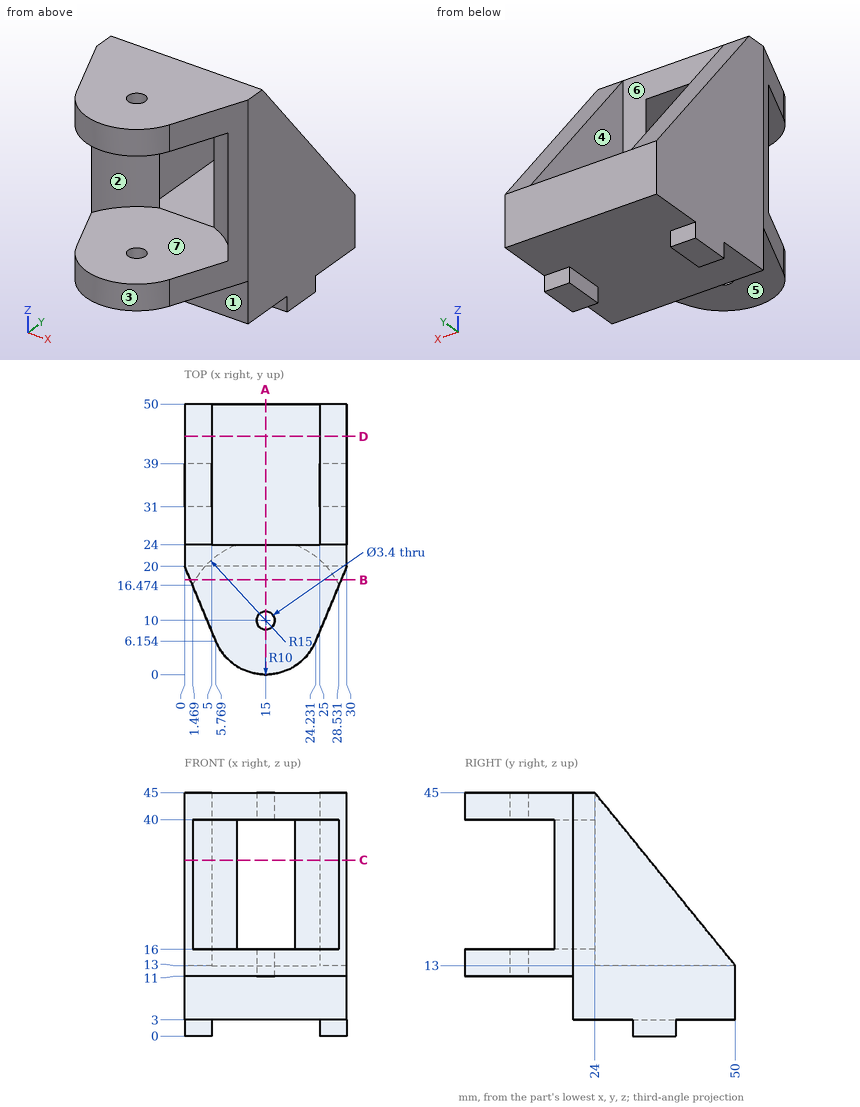
Verification items for this drawing (mm, ordinates from the low corner). A direction names the side the tool comes from. Give positions to 0.01 mm unless a question says otherwise; leave off trailing zeros. Loops run counter-clockwise (first coordinate to the right, second up) from the corner with the lowest first, then second, coordinate; pieces in that order, holes last. Notation, with made-up numbers: M -35,20 L 0,20 A14 cw 0,46 Z; hole C 75,49 d10. An arc over 180 degrees is marked long. Write item = value, one per line. Start each with the question number.
1. Section check A-A, the plane x = 15. Enter the section's corners in (y, z).
2. Section check B-B, the plane y = 17.5. Enter the section's corners in (x, z).
3. Draft check along X on the marked faces 1, 2, 3 and 4. Enter one of: +X half, -X half, draft (parallel to the pull), parting line (faces both ways), or undercut.
4. Tool access check on the marked faces 5, 6 and 7. Record the directions out of +Z, -Z, +X, -X, +Y, -Y that give a thin tool (end or side, any length) a straight path to the whole face; none if there is none.
5. Go/stop test with flat-tipped pins: P1, Ø3.5, axis at x = 27.5, z = 2, coming from the -Y side; P2, Ø12, axis at x = 23, y = 6.5, coming from the -Z side; P3, Ø0.9, axis at x = 27.5, z = 2, coming from the +Y side. Record where each tip stops, or that it passes through.
6. Thickness scan on probe 1 along Z at (x, y) = (21, 10); probe 2 along X at (y, z) = (32, 25); probe 3 along Y at (x, z) = (15, 41.4). Record the ranges inside material, lowest first.
7. Section check C-C, the plane z = 32.5. Enter the section's corners in (x, y) (1 decimal).
8. Section check D-D, the plane y = 44. Enter the section's corners in (x, z) (1 decimal), plus the area to 3 significant figures.
Values follow:
q1.outline = M 0,11 L 8.3,11 L 8.3,16 L 0,16 Z; M 0,40 L 8.3,40 L 8.3,45 L 0,45 Z; M 11.7,11 L 20,11 L 20,3 L 50,3 L 50,13 L 24,13 L 24,16 L 11.7,16 Z; M 11.7,40 L 24,40 L 24,45 L 11.7,45 Z
q2.outline = M 1.04,11 L 28.96,11 L 28.96,45 L 1.04,45 Z; hole M 2.01,16 L 27.99,16 L 27.99,40 L 2.01,40 Z
q3.face_1 = draft
q3.face_2 = undercut
q3.face_3 = parting line
q3.face_4 = undercut
q4.face_5 = -Z, +X, -X, -Y
q4.face_6 = +Z, +Y
q4.face_7 = -Y
q5.P1 = 20
q5.P2 = 11
q5.P3 = 39
q6.probe_1 = 11 to 16, 40 to 45
q6.probe_2 = 0 to 5, 25 to 30
q6.probe_3 = 0 to 8.3, 11.7 to 24
q7.outline = M 0,20 L 1.5,16.5 A15 cw 9.6,24 L 5,24 L 5,34.2 L 0,34.2 Z; M 20.4,24 A15 cw 28.5,16.5 L 30,20 L 30,34.2 L 25,34.2 L 25,24 Z
q8.outline = M 0,3 L 30,3 L 30,20.4 L 25,20.4 L 25,13 L 5,13 L 5,20.4 L 0,20.4 Z
q8.area = 374 mm^2
